```python
from build123d import *

# Parameters (mm, degrees)
BOSS_EXTRUDE1_DEPTH  = 8.636
SKETCH2_R            = 16.383
BOSS_EXTRUDE2_DEPTH  = 8.89
SKETCH5_R            = 15.494
BOSS_EXTRUDE3_DEPTH  = 22.225
SKETCH6_R            = 13.081
BOSS_EXTRUDE4_DEPTH  = 6.35
BOSS_EXTRUDE5_DEPTH  = 8.89
SKETCH19_R           = 8.509
BOSS_EXTRUDE9_DEPTH  = 20.574
SKETCH26_R           = 9.144
CUT_EXTRUDE1_DEPTH   = 55.991
SKETCH28_W           = 39.116
SKETCH28_H           = 30.48
BOSS_EXTRUDE11_DEPTH = 9.525
SKETCH29_W           = 64.008
SKETCH29_H           = 49.53
BOSS_EXTRUDE12_DEPTH = 44.45
BOSS_EXTRUDE13_DEPTH = 6.35
CUT_EXTRUDE2_REACH   = 99.689
BOSS_EXTRUDE14_DEPTH = 44.45


with BuildPart() as part:
    # Sketch1 → Boss-Extrude1 (new body)
    with BuildSketch(Plane(origin=(0, 0, 0), x_dir=(1, 0, 0), z_dir=(0, 1, 0))):
        Polygon((3.618323339, -5.199254385), (5.90723301, 10.02760322), (-6.13515766, 19.623285945), (-20.466458001, 13.992111064), (-22.755367672, -1.234746541), (-10.712977002, -10.830429265), align=None)
    extrude(amount=BOSS_EXTRUDE1_DEPTH)

    # Sketch2 → Boss-Extrude2 (add)
    with BuildSketch(Plane(origin=(0, 8.636, 0), x_dir=(1, 0, 0), z_dir=(0, 1, 0))):
        with Locations((-8.116287221, 4.517363885)):
            Circle(SKETCH2_R)
    extrude(amount=BOSS_EXTRUDE2_DEPTH)

    # Sketch5 → Boss-Extrude3 (add)
    with BuildSketch(Plane(origin=(0, 17.526, 0), x_dir=(1, 0, 0), z_dir=(0, 1, 0))):
        with Locations((-8.116287221, 4.517363885)):
            Circle(SKETCH5_R)
    extrude(amount=BOSS_EXTRUDE3_DEPTH)

    # Sketch6 → Boss-Extrude4 (add)
    with BuildSketch(Plane(origin=(0, 39.751, 0), x_dir=(1, 0, 0), z_dir=(0, 1, 0))):
        with Locations((-8.116287221, 4.517363885)):
            Circle(SKETCH6_R)
    extrude(amount=BOSS_EXTRUDE4_DEPTH)

    # Sketch8 → Boss-Extrude5 (add)
    with BuildSketch(Plane(origin=(0, 46.101, 0), x_dir=(1, 0, 0), z_dir=(0, 1, 0))):
        Polygon((-18.441823617, 15.940130543), (-23.171461527, 1.286570387), (-12.845925131, -10.136196271), (2.209249175, -6.905402773), (6.938887085, 7.748157383), (-3.386649312, 19.170924041), align=None)
    extrude(amount=BOSS_EXTRUDE5_DEPTH)

    # Sketch19 → Boss-Extrude9 (add)
    with BuildSketch(Plane(origin=(-5.896918877, 0, -6.523547615), x_dir=(-0.741837728, 0, 0.67057944), z_dir=(-0.67057944, 0, -0.741837728))):
        with Locations((2.991716732, 28.575)):
            Circle(SKETCH19_R)
    extrude(amount=BOSS_EXTRUDE9_DEPTH)

    # Sketch26 → Cut-Extrude1 (cut, through all)
    with BuildSketch(Plane(origin=(0, 54.991, 0), x_dir=(1, 0, 0), z_dir=(0, 1, 0))):
        with Locations((-8.116287221, 4.517363885)):
            Circle(SKETCH26_R)
    extrude(amount=-CUT_EXTRUDE1_DEPTH, mode=Mode.SUBTRACT)

    # Sketch28 → Boss-Extrude11 (add)
    with BuildSketch(Plane(origin=(-19.693420267, 0, -21.786117038), x_dir=(-0.741837728, 0, 0.67057944), z_dir=(-0.67057944, 0, -0.741837728))):
        with Locations((2.991716732, 28.575)):
            Rectangle(SKETCH28_W, SKETCH28_H)
    extrude(amount=BOSS_EXTRUDE11_DEPTH)

    # Sketch29 → Boss-Extrude12 (add)
    with BuildSketch(Plane(origin=(-26.080689429, 0, -28.852121401), x_dir=(-0.741837728, 0, 0.67057944), z_dir=(-0.67057944, 0, -0.741837728))):
        with Locations((12.389716732, 33.401)):
            Rectangle(SKETCH29_W, SKETCH29_H)
    extrude(amount=BOSS_EXTRUDE12_DEPTH)

    # Sketch31 → Boss-Extrude13 (add)
    with BuildSketch(Plane(origin=(-26.080689429, 0, -28.852121401), x_dir=(0.741837728, 0, -0.67057944), z_dir=(0.67057944, 0, 0.741837728))):
        Polygon((-29.660890196, 11.58925085), (-25.479774792, 15.49154325), (-26.768701441, 21.063641607), (-32.238743495, 22.733447563), (-36.419858899, 18.831155162), (-35.130932249, 13.259056806), align=None)
    extrude(amount=BOSS_EXTRUDE13_DEPTH)

    # Sketch36 → Cut-Extrude2 (cut, up to next)
    with BuildSketch(Plane(origin=(-55.887945518, 0, -61.826808426), x_dir=(-0.741837728, 0, 0.67057944), z_dir=(-0.67057944, 0, -0.741837728)), mode=Mode.PRIVATE) as cut_extrude2_sk1:
        Polygon((34.233716732, 8.636), (44.393716732, 18.796), (44.393716732, 8.636), align=None)
    cut_extrude2_tool1 = extrude(cut_extrude2_sk1.sketch, amount=-CUT_EXTRUDE2_REACH, mode=Mode.PRIVATE) & part.part
    add(cut_extrude2_tool1.solids().sort_by_distance((-86.308522, 12.022667, -34.328324))[0], mode=Mode.SUBTRACT)
    # Sketch36 → Cut-Extrude2 (cut, up to next)
    with BuildSketch(Plane(origin=(-55.887945518, 0, -61.826808426), x_dir=(-0.741837728, 0, 0.67057944), z_dir=(-0.67057944, 0, -0.741837728)), mode=Mode.PRIVATE) as cut_extrude2_sk2:
        Polygon((-9.454283268, 8.636), (-19.614283268, 18.796), (-19.614283268, 8.636), align=None)
    cut_extrude2_tool2 = extrude(cut_extrude2_sk2.sketch, amount=-CUT_EXTRUDE2_REACH, mode=Mode.PRIVATE) & part.part
    add(cut_extrude2_tool2.solids().sort_by_distance((-43.849687, 12.022667, -72.708714))[0], mode=Mode.SUBTRACT)
    # Sketch36 → Cut-Extrude2 (cut, up to next)
    with BuildSketch(Plane(origin=(-55.887945518, 0, -61.826808426), x_dir=(-0.741837728, 0, 0.67057944), z_dir=(-0.67057944, 0, -0.741837728)), mode=Mode.PRIVATE) as cut_extrude2_sk3:
        Polygon((-19.614283268, 48.006), (-9.454283268, 58.166), (-19.614283268, 58.166), align=None)
    cut_extrude2_tool3 = extrude(cut_extrude2_sk3.sketch, amount=-CUT_EXTRUDE2_REACH, mode=Mode.PRIVATE) & part.part
    add(cut_extrude2_tool3.solids().sort_by_distance((-43.849687, 54.779333, -72.708714))[0], mode=Mode.SUBTRACT)
    # Sketch36 → Cut-Extrude2 (cut, up to next)
    with BuildSketch(Plane(origin=(-55.887945518, 0, -61.826808426), x_dir=(-0.741837728, 0, 0.67057944), z_dir=(-0.67057944, 0, -0.741837728)), mode=Mode.PRIVATE) as cut_extrude2_sk4:
        Polygon((44.393716732, 48.006), (34.233716732, 58.166), (44.393716732, 58.166), align=None)
    cut_extrude2_tool4 = extrude(cut_extrude2_sk4.sketch, amount=-CUT_EXTRUDE2_REACH, mode=Mode.PRIVATE) & part.part
    add(cut_extrude2_tool4.solids().sort_by_distance((-86.308522, 54.779333, -34.328324))[0], mode=Mode.SUBTRACT)

    # Sketch37 → Boss-Extrude14 (add)
    with BuildSketch(Plane(origin=(-55.887945518, 0, -61.826808426), x_dir=(-0.741837728, 0, 0.67057944), z_dir=(-0.67057944, 0, -0.741837728))):
        with BuildLine():
            Line((42.007793569, 16.410076836), (36.619639896, 11.021923164))
            ThreePointArc((36.619639896, 11.021923164), (42.007793569, 11.021923164), (42.007793569, 16.410076836))
        make_face()
        with BuildLine():
            Line((-11.840206431, 11.021923164), (-17.228360104, 16.410076836))
            ThreePointArc((-17.228360104, 16.410076836), (-17.228360104, 11.021923164), (-11.840206431, 11.021923164))
        make_face()
        with BuildLine():
            Line((-17.228360104, 50.391923164), (-11.840206431, 55.780076836))
            ThreePointArc((-11.840206431, 55.780076836), (-17.228360104, 55.780076836), (-17.228360104, 50.391923164))
        make_face()
        with BuildLine():
            Line((36.619639896, 55.780076836), (42.007793569, 50.391923164))
            ThreePointArc((42.007793569, 50.391923164), (42.007793569, 55.780076836), (36.619639896, 55.780076836))
        make_face()
    extrude(amount=-BOSS_EXTRUDE14_DEPTH)


solid = part.part
```
CAD build for the part. Positions are in the model's coordinates, mm. A direction names the side the tool comes from. Round coordinates to 2 decimals unless told otherwise and drop trailing zeros. Order: outer loops, then holes, each group sorted by start corner. A loop starts at its lowest first (then second) coordinate and runs counter-clockwise, first axis right, second up.
Item 1: Saw through at A-A on y = 26. Write the cut outline in (x, z), then the cut area to 3 significant figures.
Item 2: Pin check, flat tips, straight feed: pin 1 (16 mm diameter, centred on x = -28.5, z = -20.5, fed in from -Y); pin 2 (10 mm diameter, centred on x = -5, z = 2, fed in from +Y); pin 3 (8 mm diameter, centred on y = 39, z = -50, fed in from -X). Stop position of each tip, or through.
Item 3: Tool access for faces 1 (the face through (-44.839, 17.239, -3.336)), 2 (the face through (-27.51, 49.18, -57.93)), 3 (the face through (-73.23, 17.59, -16.61)), 4 (the face through (4.54, 50.48, -0.32)): list every direction of +Z, -Z, +X, -X, +Y, -Y with a clear straight run to the whole face (end or side of a thin tool).
Item 4: Mould opens along Y. For faces 5 (the face through (-73.253, 49.182, -16.59)), 6 (the face through (-67.46, 9.81, -21.83)), 7 (the face through (-16.818, 4.258, 5.965)) say: pulls with the +Y half, pulls with the -Y half, needs draft (parallel to the pull), parting line crosses it, or undercut.
Item 5: Probe line 1 along X through (y, z) = (27.5, -13); line 2 along Z through (x, y) = (-7.5, 23); line 3 along Y through (x, z) = (-62, -35). List the from-to ranges inside material, lowest first.
Reported:
1. outline: (-88.82, -32.06) - (-41.34, -74.98) - (-11.53, -42.01) - (-13.79, -39.96) - (-7.4, -32.9) - (-15.9, -25.22) - (-10.95, -19.75) arc R15.49 ccw (long way) to (-22.99, -8.87) - (-27.93, -14.34) - (-36.42, -6.66) - (-42.81, -13.73) - (-59.01, 0.92) - close; hole circle Ø18.29 at (-8.12, -4.52)
1. area: 3,800 mm2
2. pin 1: stops at y = 8.64
2. pin 2: stops at y = 54.99
2. pin 3: stops at x = -73.4
3. face 1: +Z, +Y, -Y
3. face 2: -Z, +X
3. face 3: +Z, -X
3. face 4: +Z, +X, +Y
4. face 5: undercut
4. face 6: pulls with the -Y half
4. face 7: needs draft
5. line 1: x = -71.59 to -43.62, -42.15 to -29.41, -27.16 to -11.53, -4.7 to 4.85
5. line 2: z = -33 to -32.81, -20 to -13.64, 4.61 to 10.96
5. line 3: y = 8.64 to 58.17
